Autodesk Inventor part; units mm, degrees
ref_plane "YZ Plane" through (0, 0, 0) normal (1, 0, 0) x (0, 1, 0)
ref_plane "XZ Plane" through (0, 0, 0) normal (0, 1, 0) x (-1, 0, 0)
ref_plane "XY Plane" through (0, 0, 0) normal (0, 0, 1) x (1, 0, 0)
sketch "Sketch1" plane through (0, 0, 0) normal (0, 1, 0) x (-1, 0, 0)
  line L0 (0, -50.8) -> (50.8, -50.8)
  line L1 (50.8, -50.8) -> (50.8, 0)
  line L2 (-50.8, 50.8) -> (50.8, -50.8) construction
  line L3 (-50.8, -50.8) -> (50.8, 50.8) construction
  line L4 (0, -28.575) -> (28.575, -28.575)
  line L5 (28.575, -28.575) -> (28.575, 0)
  line L6 (-28.575, 28.575) -> (28.575, -28.575) construction
  line L7 (-28.575, -28.575) -> (28.575, 28.575) construction
  line L8 (50.8, 0) -> (28.575, 0)
  line L9 (0, -28.575) -> (0, -50.8)
  point P0 (0, 0)
  dimension "d2" = 50.8
extrude "Extrusion1" add sketch "Sketch1" along normal blind 1365.25
properties part number "Molding 4 ft 5 3_4 in"
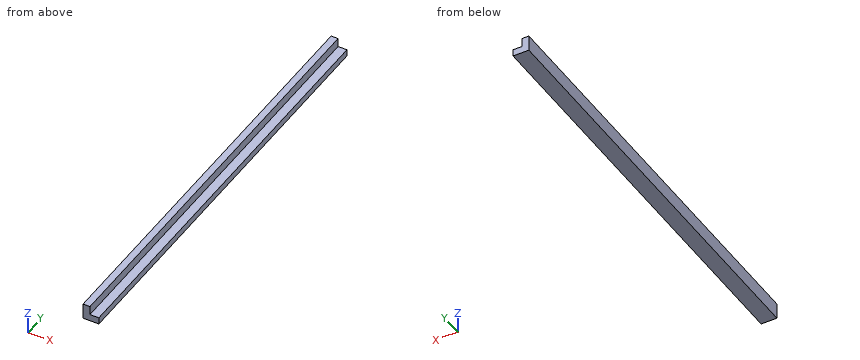
CAD build for the part. Positions are in the model's coordinates, mm. Give positions to 0.01 mm unless a question says otherwise; leave off trailing zeros. Order: outer loops, then holes, each group sorted by start corner. A loop starts at its lowest first (then second) coordinate and runs counter-clockwise, first axis right, second up. Notation, with made-up numbers: (29.25, 29.5) - (57.25, 29.5) arc R20 ccw to (57.25, 41.5) - close; hole circle Ø2 at (74.25, 9). An arc over 180 degrees is marked (long way). Write each question's results on one line, items separated by ' | '.
1. Probe L1, parallel to X at y = 670, z = -3 (3 decimals). List the from-to ranges inside material, lowest first. Write a range as from..to.
Calculated:
L1: x = -50.8..-28.575
2. Saw through at A-A on x = -19. List the corners of the cut face in (y, z) (3 decimals), and give its area (3 significant figures).
Calculated:
outline: (0, -50.8) - (1365.25, -50.8) - (1365.25, -28.575) - (0, -28.575) - close | area: 30,300 mm2
3. Pin check, flat tips, straight feed: pin 1 (23 mm diameter, centred on x = -12.5, y = 1010.5, fed in from +Z) (3 decimals); pin 2 (8.5 mm diameter, centred on y = 434.5, z = -16, fed in from +X) (3 decimals). Stop position of each tip, or through.
Calculated:
pin 1: stops at z = -28.575 | pin 2: stops at x = -28.575
4. Saw through at C-C on z = -14.5. List the corners of the cut face in (x, y) (3 decimals), and give its area (3 significant figures).
Calculated:
outline: (-50.8, 0) - (-28.575, 0) - (-28.575, 1365.25) - (-50.8, 1365.25) - close | area: 30,300 mm2
5. Saw through at B-B on y = 610. List the corners of the cut face in (x, z) (3 decimals).
Calculated:
outline: (-50.8, -50.8) - (0, -50.8) - (0, -28.575) - (-28.575, -28.575) - (-28.575, 0) - (-50.8, 0) - close
